Autodesk Inventor part; units mm, degrees
ref_plane "YZ Plane" through (0, 0, 0) normal (1, 0, 0) x (0, 1, 0)
ref_plane "XZ Plane" through (0, 0, 0) normal (0, 1, 0) x (-1, 0, 0)
ref_plane "XY Plane" through (0, 0, 0) normal (0, 0, 1) x (1, 0, 0)
sketch "Sketch1" plane through (0, 0, 0) normal (0, 1, 0) x (-1, 0, 0)
  line L0 (-100, 30) -> (100, 30)
  line L1 (100, 30) -> (100, -30)
  line L2 (100, -30) -> (-100, -30)
  line L3 (-100, -30) -> (-100, 30)
  circle A0 centre (60, 14) radius 2
  circle A1 centre (31, 14) radius 2
  circle A2 centre (-31, 14) radius 2
  circle A3 centre (-60, 14) radius 2
  circle A4 centre (20, 12) radius 2
  circle A5 centre (-20, 12) radius 2
  circle A6 centre (60, -4.55) radius 2
  circle A7 centre (31, -4.55) radius 2
  circle A8 centre (20, -12) radius 2
  circle A9 centre (-20, -12) radius 2
  circle A10 centre (-31, -4.55) radius 2
  circle A11 centre (-60, -4.55) radius 2
  point P0 (0, 0)
  dimension "d0" = 200
  dimension "d1" = 60
  dimension "d7" = 4
  dimension "d12" = 4
  dimension "d15" = 4
  dimension "d16" = 4
  dimension "d18" = 4
  dimension "d19" = 4
  dimension "d23" = 4
  dimension "d24" = 4
  dimension "d25" = 18.55
  dimension "d30" = 100
extrude "Extrusion1" add sketch "Sketch1" along normal blind 9.525 contours L0 L1 L2 L3 | A10 | A11
fillet "Fillet1" radius 4 4 edges at (100, 4.7625, -30) (-100, 4.7625, -30) (100, 4.7625, 30) (-100, 4.7625, 30)
sketch "Sketch2" plane through (0, 9.525, 0) normal (0, 1, 0) x (1, 0, 0)
  circle A0 centre (31, -14) radius 2
  circle A1 centre (60, -14) radius 2
  circle A2 centre (31, 4.55) radius 2
  circle A3 centre (60, 4.55) radius 2
  point P0 (0, 0)
  dimension "d26" = 4
  dimension "d27" = 4
extrude "Extrusion2" cut sketch "Sketch2" against normal blind 9.525 contours A2 | A3
properties part number "Placa Herramienta"
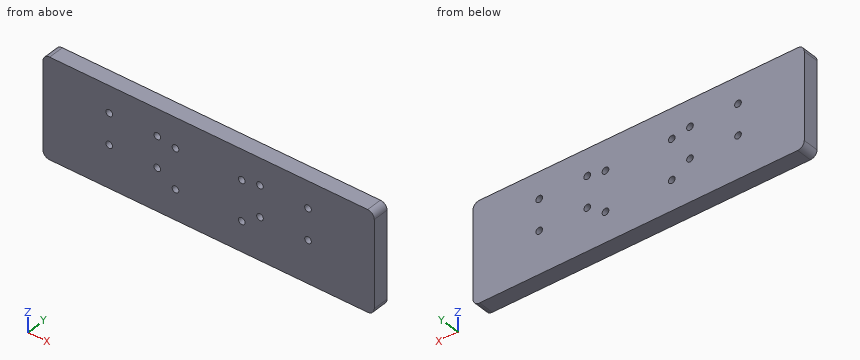
Read the model definition and answer for the solid it produces. Units are mm, in the model's axes. Coordinates: 2 decimals unless noted, no trailing zeros. Order: outer loops, then holes, each group sorted by start corner. A loop starts at its lowest first (then second) coordinate and runs counter-clockwise, first axis right, second up. Notation, with made-up numbers: M 65.5,28.25 L 84.5,28.25 A21 cw 84.5,59.25 Z; hole C 79.25,66.5 d10. An arc over 180 degrees is marked long. Put each result on its own line as item: value. Start each with the question number.
Item 1: Consider probe 1 along Z at (x, y) = (20, 3); probe 2 along Z at (x, y) = (-31, 4.5); probe 3 along X at (y, z) = (4, -5). Determine where each line is inside the solid, lowest interval first. Write a range as [from, to].
Item 2: Section B-B, the plane z = -12 is taken. Determine the outline of the cut face in (x, y) (3 decimals).
Item 3: Section A-A, the plane x = 20 is taken. Determine the outline of the cut face in (y, z) (3 decimals).
Computed:
1. probe 1: z = [-30, -14], [-10, 10], [14, 30]
1. probe 2: z = [-30, -6.55], [-2.55, 12], [16, 30]
1. probe 3: x = [-100, -61.95], [-58.05, -32.95], [-29.05, 29.05], [32.95, 58.05], [61.95, 100]
2. outline: M -100,0 L -22,0 L -22,9.525 L -100,9.525 Z; M -18,0 L 18,0 L 18,9.525 L -18,9.525 Z; M 22,0 L 100,0 L 100,9.525 L 22,9.525 Z
3. outline: M 0,-30 L 9.525,-30 L 9.525,-14 L 0,-14 Z; M 0,-10 L 9.525,-10 L 9.525,10 L 0,10 Z; M 0,14 L 9.525,14 L 9.525,30 L 0,30 Z
